CAD build for the part. Positions are in the model's coordinates, mm. A direction names the side the tool comes from. Give positions to 0.01 mm unless a question says otherwise; leave off trailing zeros. Loops run counter-clockwise (first coordinate to the right, second up) from the corner with the lowest first, then second, coordinate; pieces in that order, holes last. Notation, with made-up numbers: M 77.25,16 L 127.25,16 A20 ccw 127.25,27 Z; hole C -40,29 d3. An arc over 180 degrees is marked long. One line per question, with ' | ' between items.
```python
from build123d import *

# Parameters (mm, degrees)
EXTRUDE_1_DEPTH     = 3
SKETCH_2_R          = 1.5
CUT_EXTRUDE_1_DEPTH = 3


with BuildPart() as part:
    # 草图1 → 凸台-拉伸1 (new body)
    with BuildSketch(Plane(origin=(0, 0, 0), x_dir=(0, 0, -1), z_dir=(1, 0, 0))):
        with BuildLine():
            Line((0, 0), (40, 0))
            Line((40, 0), (40, -15))
            Line((40, -15), (32.5, -15))
            ThreePointArc((32.5, -15), (28.964466094, -16.464466094), (27.5, -20))
            Line((27.5, -20), (27.5, -45))
            Line((27.5, -45), (12.5, -45))
            Line((12.5, -45), (12.5, -20))
            ThreePointArc((12.5, -20), (11.035533906, -16.464466094), (7.5, -15))
            Line((7.5, -15), (0, -15))
            Line((0, -15), (0, 0))
        make_face()
    extrude(amount=EXTRUDE_1_DEPTH)

    # 草图2 → 切除-拉伸1 (cut)
    with BuildSketch(Plane(origin=(3, 0, 0), x_dir=(0, 0, -1), z_dir=(1, 0, 0))):
        with Locations((31, -7.5)):
            Circle(SKETCH_2_R)
        with Locations((9, -7.5)):
            Circle(SKETCH_2_R)
        with Locations((20, -39)):
            Circle(SKETCH_2_R)
        with Locations((20, -24)):
            Circle(SKETCH_2_R)
    extrude(amount=-CUT_EXTRUDE_1_DEPTH, mode=Mode.SUBTRACT)


solid = part.part
```
Item 1: Drill centre lines: line 1 along Y through (x, z) = (2, -20); line 2 along Z through (x, y) = (1.7, -6.5); line 3 along Y through (x, z) = (0.4, -1.5). Where is each one in solid material? Low to high. Write a range as [from, to].
Conclusion:
line 1: [-45, -40.5], [-37.5, -25.5], [-22.5, 0] | line 2: [-40, -32.12], [-29.88, -10.12], [-7.88, 0] | line 3: [-15, 0]
Item 2: Saw through at C-C on y = -39. Give the cut face in (x, z), and give its area (3 significant figures).
Conclusion:
outline: M 0,-27.5 L 3,-27.5 L 3,-21.5 L 0,-21.5 Z; M 0,-18.5 L 3,-18.5 L 3,-12.5 L 0,-12.5 Z | area: 36.0 mm²
Item 3: Saw through at B-B on x = 2.3. Give the cut face in (y, z).
Conclusion:
outline: M -45,-27.5 L -20,-27.5 A5 cw -15,-32.5 L -15,-40 L 0,-40 L 0,0 L -15,0 L -15,-7.5 A5 cw -20,-12.5 L -45,-12.5 Z; hole C -39,-20 d3; hole C -24,-20 d3; hole C -7.5,-31 d3; hole C -7.5,-9 d3
Item 4: 3-axis set-ups, long thin cutter, end or side, ignore diameter. For faces 4 (the flat face through (1, -15, -4)), 5 (the flat face through (1, -15, -36)), 6 (the cylindrical face through (1.52, -7.43, -29.5)): which of +Z, -Z, +X, -X, +Y, -Y reach the whole face in a straight line?
Conclusion:
face 4: +Z, +X, -X, -Y | face 5: -Z, +X, -X, -Y | face 6: +X, -X
Item 5: Saw through at A-A on z = -20. Give the cut face in (x, y), and give its area (3 significant figures).
Conclusion:
outline: M 0,-45 L 3,-45 L 3,-40.5 L 0,-40.5 Z; M 0,-37.5 L 3,-37.5 L 3,-25.5 L 0,-25.5 Z; M 0,-22.5 L 3,-22.5 L 3,0 L 0,0 Z | area: 117 mm²
Item 6: Mould opens along Z. For faces 1 (the cylindrical face through (1.5, -39.9, -18.8)), 2 (the flat face through (1, -33, -12.5)), 3 (the flat face through (1, -32, -27.5)) say: pulls with the +Z half, pulls with the -Z half, needs draft (parallel to the pull), parting line crosses it, or undercut.
Conclusion:
face 1: undercut | face 2: pulls with the +Z half | face 3: pulls with the -Z half
Item 7: Saw through at D-D on y = -7.5. Give the cut face in (x, z).
Conclusion:
outline: M 0,-40 L 3,-40 L 3,-32.5 L 0,-32.5 Z; M 0,-29.5 L 3,-29.5 L 3,-10.5 L 0,-10.5 Z; M 0,-7.5 L 3,-7.5 L 3,0 L 0,0 Z
Item 8: Drop flat-ended pins along their axis: P1, Ø1.5, axis at x = 1, y = -32, coming from the -Z side; P2, Ø4, axis at y = -24, z = -20, coming from the +X side; P3, Ø1.5, axis at x = 1.5, z = -4.5, coming from the -Y side; P4, Ø1.5, axis at x = 1, y = -28, coming from the +Z side. Give the stop position or say it passes through.
Conclusion:
P1: z = -27.5 | P2: x = 3 | P3: y = -15 | P4: z = -12.5
